```python
from build123d import *

# Parameters (mm, degrees)
F0_W     = 101.6
F0_H     = 25.4
F1_DEPTH = 9.525


with BuildPart() as f1:
    # F0 (on Top) → F1 (new body)
    with BuildSketch(Plane.XY):
        Polygon((-157.645054, 179.173873), (-175.267478, 161.506097), (-179.751833, 157.010203), (-22.079604, -0.257338), (-179.347144, -157.929566), (-174.851251, -162.413921), (-157.183479, -180.03635), (-152.693351, -184.526479), (12.783127, -19.05), (238.290359, -19.05), (238.290359, -12.7), (238.290359, 12.7), (238.290359, 19.05), (12.307383, 19.05), (-153.16648, 183.675526), align=None)
        Polygon((-165.882541, -153.422133), (-94.344681, -81.276558), (-76.361107, -99.213979), (-148.214769, -171.044564), align=None, mode=Mode.SUBTRACT)
        Polygon((-67.180604, -90.433441), (-85.164157, -72.496041), (-13.101294, -0.875487), (-85.349598, 71.819004), (-67.412202, 89.802561), (9.690359, 12.7), (111.290359, 12.7), (111.290359, -12.7), (10.552837, -12.7), align=None, mode=Mode.SUBTRACT)
        Polygon((-76.61524, 98.559477), (-94.552657, 80.575898), (-166.27569, 152.537388), (-148.653264, 170.205165), align=None, mode=Mode.SUBTRACT)
        with Locations((174.790359, 0)):
            Rectangle(F0_W, F0_H, mode=Mode.SUBTRACT)
    extrude(amount=F1_DEPTH)


solid = f1.part
```
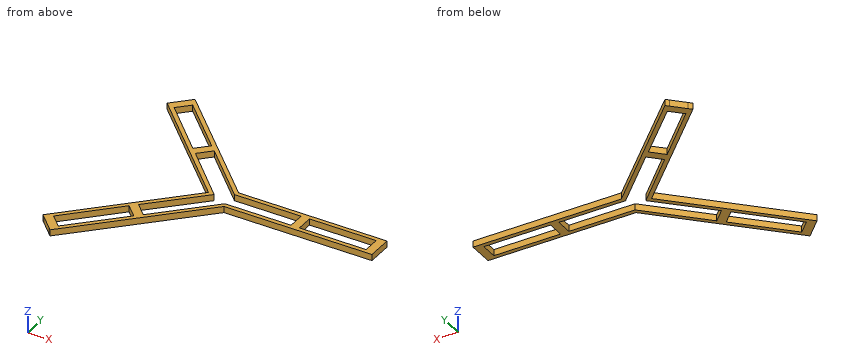
Work out the finished part from the listing and answer in its coordinate system (mm). Give positions to 0.01 mm unless a question says otherwise; leave off trailing zeros. Write each loop counter-clockwise with the first axis right and the second up, starting at its lowest first coordinate (ties: lowest second). Pieces come first, ordered by that corner, then holes. Notation, with made-up numbers: (87.25, -40) -> (135.25, -40) arc R18 cw to (135.25, -19) -> close; hole circle Ø5 at (-10, 61.5). An arc over 180 degrees is marked (long way). Write item = value, one per line.
Q1. Section D-D on x = -132 is taken. Determine the outline of the cut face in (y, z) (3 decimals), and give its area (3 significant figures).
Computed values:
outline = (-163.833, 0) -> (-154.835, 0) -> (-154.835, 9.525) -> (-163.833, 9.525) -> close; (-119.252, 0) -> (-110.461, 0) -> (-110.461, 9.525) -> (-119.252, 9.525) -> close; (109.381, 0) -> (118.148, 0) -> (118.148, 9.525) -> (109.381, 9.525) -> close; (153.643, 0) -> (162.618, 0) -> (162.618, 9.525) -> (153.643, 9.525) -> close
area = 338 mm^2
Q2. Section B-B on x = 62.5 is taken. Determine the outline of the cut face in (y, z) (3 decimals).
Computed values:
outline = (-19.05, 0) -> (-12.7, 0) -> (-12.7, 9.525) -> (-19.05, 9.525) -> close; (12.7, 0) -> (19.05, 0) -> (19.05, 9.525) -> (12.7, 9.525) -> close
Q3. Section A-A on z = 3.25 is taken. State how many separate pieces and enclosed holes the cut face has, and give its area (3 significant figures).
Computed values:
separate_pieces = 1
enclosed_holes = 4
area = 10,600 mm^2
Q4. Consider line 1 along Y through (x, z) = (22.5, 5); line 2 along X through (y, z) = (-9, 4.75); line 3 along Y through (x, z) = (-73, 2.5). Determine where each line is inside the solid, lowest interval first.
Computed values:
line_1 = -19.05 to -12.7, 12.7 to 19.05
line_2 = -30.8 to -21.28, 111.29 to 123.99, 225.59 to 238.29
line_3 = -104.83 to -84.63, -60.41 to -51.31, 50.53 to 59.39, 84.2 to 103.92
Q5. Section C-C on y = -36.5 is taken. Determine the outline of the cut face in (x, z) (3 decimals).
Computed values:
outline = (-58.229, 0) -> (-48.946, 0) -> (-48.946, 9.525) -> (-58.229, 9.525) -> close; (-13.247, 0) -> (-4.667, 0) -> (-4.667, 9.525) -> (-13.247, 9.525) -> close
Q6. Flat-ended cylindrical pins translate along their axes: pin 1 Ø1.5 at (y, z) = (22.5, 4.5) entering from -X; pin 2 Ø5 at (y, z) = (6, 6) entering from -X; pin 3 Ø3 at (y, z) = (2, 5.5) entering from -X; pin 4 Ø3 at (x, y) = (146.5, -10.5) entering from -Z. Find the tip coordinate at first contact, or state that the pin passes through.
Computed values:
pin_1 = -45.65
pin_2 = -30.86
pin_3 = -25.85
pin_4 = through
